from build123d import *

# Parameters (mm, degrees)
SKETCH1_W            = 98.425
SKETCH1_H            = 12.7
BOSS_EXTRUDE1_DEPTH  = 12.7
CUT_EXTRUDE1_REACH   = 54.388
SKETCH2_W            = 6.35
SKETCH2_H            = 19.05
FILLET1_R            = 3.175
FILLET2_R            = 3.175
FILLET3_R            = 3.175
FILLET4_R            = 3.175
FILLET1_OF_MIRROR1_R = 3.175
FILLET2_OF_MIRROR1_R = 3.175
FILLET3_OF_MIRROR1_R = 3.175
FILLET4_OF_MIRROR1_R = 3.175
CUT_EXTRUDE2_REACH   = 54.388
SKETCH5_W            = 55.88
SKETCH5_H            = 12.7
SKETCH6_W            = 25.4
SKETCH6_H            = 50.8
BOSS_EXTRUDE3_DEPTH  = 6.35


with BuildPart() as part:
    # Sketch1 → Boss-Extrude1 (new, symmetric)
    with BuildSketch(Plane.XY):
        Rectangle(SKETCH1_W, SKETCH1_H)
    extrude(amount=BOSS_EXTRUDE1_DEPTH, both=True)

    # Sketch2 → Cut-Extrude1 (cut, up to next)
    with BuildSketch(Plane(origin=(0, 6.35, 0), x_dir=(1, 0, 0), z_dir=(0, 1, 0)), mode=Mode.PRIVATE) as cut_extrude1_sk1:
        with Locations((-41.275, 0)):
            Rectangle(SKETCH2_W, SKETCH2_H)
    cut_extrude1_tool1 = extrude(cut_extrude1_sk1.sketch, amount=-CUT_EXTRUDE1_REACH, mode=Mode.PRIVATE) & part.part
    cut_extrude1 = cut_extrude1_tool1.solids().sort_by_distance((-41.275, 6.35, 0))[0]
    add(cut_extrude1, mode=Mode.SUBTRACT)

    # Fillet1
    fillet1_edges = [part.edges().sort_by_distance(p)[0] for p in [
        (-44.45, 0, -9.525),
    ]]
    fillet(fillet1_edges, radius=FILLET1_R)

    # Fillet2
    fillet2_edges = [part.edges().sort_by_distance(p)[0] for p in [
        (-38.1, 0, -9.525),
    ]]
    fillet(fillet2_edges, radius=FILLET2_R - 0.0001)  # a hair under: the kernel refuses the full size

    # Fillet3
    fillet3_edges = [part.edges().sort_by_distance(p)[0] for p in [
        (-44.45, 0, 9.525),
    ]]
    fillet(fillet3_edges, radius=FILLET3_R)

    # Fillet4
    fillet4_edges = [part.edges().sort_by_distance(p)[0] for p in [
        (-38.1, 0, 9.525),
    ]]
    fillet(fillet4_edges, radius=FILLET4_R - 0.0001)  # a hair under: the kernel refuses the full size

    # Mirror1: Cut-Extrude1 across plane
    add(cut_extrude1.mirror(Plane(origin=(0, 0, 0), x_dir=(0, 0, 1), z_dir=(1, 0, 0))), mode=Mode.SUBTRACT)

    # Fillet1 of Mirror1
    fillet1_of_mirror1_edges = [part.edges().sort_by_distance(p)[0] for p in [
        (44.45, 0, -9.525),
    ]]
    fillet(fillet1_of_mirror1_edges, radius=FILLET1_OF_MIRROR1_R)

    # Fillet2 of Mirror1
    fillet2_of_mirror1_edges = [part.edges().sort_by_distance(p)[0] for p in [
        (38.1, 0, -9.525),
    ]]
    fillet(fillet2_of_mirror1_edges, radius=FILLET2_OF_MIRROR1_R - 0.0001)  # a hair under: the kernel refuses the full size

    # Fillet3 of Mirror1
    fillet3_of_mirror1_edges = [part.edges().sort_by_distance(p)[0] for p in [
        (44.45, 0, 9.525),
    ]]
    fillet(fillet3_of_mirror1_edges, radius=FILLET3_OF_MIRROR1_R)

    # Fillet4 of Mirror1
    fillet4_of_mirror1_edges = [part.edges().sort_by_distance(p)[0] for p in [
        (38.1, 0, 9.525),
    ]]
    fillet(fillet4_of_mirror1_edges, radius=FILLET4_OF_MIRROR1_R - 0.0001)  # a hair under: the kernel refuses the full size

    # Sketch5 → Cut-Extrude2 (cut, up to next)
    with BuildSketch(Plane(origin=(0, 6.35, 0), x_dir=(1, 0, 0), z_dir=(0, 1, 0)), mode=Mode.PRIVATE) as cut_extrude2_sk1:
        with Locations((0, 6.35)):
            Rectangle(SKETCH5_W, SKETCH5_H)
    cut_extrude2_tool1 = extrude(cut_extrude2_sk1.sketch, amount=-CUT_EXTRUDE2_REACH, mode=Mode.PRIVATE) & part.part
    add(cut_extrude2_tool1.solids().sort_by_distance((0, 6.35, -6.35))[0], mode=Mode.SUBTRACT)

    # Sketch6 → Boss-Extrude3 (add)
    with BuildSketch(Plane(origin=(0, 0, 0), x_dir=(-1, 0, 0), z_dir=(0, 0, -1))):
        Rectangle(SKETCH6_W, SKETCH6_H)
    extrude(amount=BOSS_EXTRUDE3_DEPTH)


solid = part.part
Design review of the part built by this model. Coordinates are the model's own, in mm. A direction names the side the tool comes from. Give positions to 0.01 mm unless a question says otherwise; leave off trailing zeros. Loops run counter-clockwise (first coordinate to the right, second up) from the corner with the lowest first, then second, coordinate; pieces in that order, holes last. Notation, with made-up numbers: (76.5, 13.5) - (126.5, 13.5) arc R16 ccw to (126.5, 17.5) - close; hole circle Ø3 at (-23, 28.5). An arc over 180 degrees is marked (long way). Use CSV: the item, a comma, the result in double quotes. Start each with the question number.
1. Machinability: for faces 1 (the flat face through (0, 16, 0)), 2 (the flat face through (-44.45, 0, 0)), 3 (the flat face through (-20, 0, 0)), which of the approach directions +Z, -Z, +X, -X, +Y, -Y give a long, thin tool a straight path to every point of the face, cutting with its end or side? Answer none if there is none.
2. Draft analysis for pull direction Z (two halves, no side actions). For faces 4 (the flat face through (0, -25.4, -3)), 5 (the flat face through (-39, 0, -12.7)), 6 (the cylindrical face through (39.055, -0.089, -8.62)), 7 (the cylindrical face through (-43.545, -0.089, 8.57)), state which applies: released by +Z, released by -Z, zero draft, split by the parting line, or undercut.
3. Add section B-B (z = -1). State the section outline as (x, y) points.
4. Add section D-D (z = -7.5). State the section outline as (x, y) points, plus the area to 3 significant figures.
5. Wall thickness on L1, parallel to X at y = -4, z = 5.75; L2, parallel to Y at x = 4, z = 4; L3, parallel to X at y = -19, z = -1.5: over which ranges is each line inside the solid? List them lowest first.
6. Add section C-C (x = -6). State the section outline as (y, z) points.
7. Add section A-A (y = 2.5). Count the separate pieces of the cut face and the enclosed holes in it, plus the area to 3 significant figures.
8. Insertion check: P1, Ø5, axis at y = 9.5, z = -2, coming from the +X side; P2, Ø12.5, axis at x = 20, z = 0.5, coming from the +Y side; P3, Ø15, axis at x = 1, y = 14, coming from the +Z side; P4, Ø2, axis at y = -9, z = 7.5, coming from the +X side. Each pin has a flat end and moves straight along its axis. Give the tip position at first contact, or say it passes through.
Results found:
1,face 1,"+Z, +X, -X, +Y"
1,face 2,"+Y, -Y"
1,face 3,"-Z, +Y, -Y"
2,face 4,"zero draft"
2,face 5,"released by -Z"
2,face 6,"undercut"
2,face 7,"undercut"
3,outline,"(-49.21, -6.35) - (-44.45, -6.35) - (-44.45, 6.35) - (-49.21, 6.35) - close; (-38.1, -6.35) - (-27.94, -6.35) - (-27.94, 6.35) - (-38.1, 6.35) - close; (-12.7, -25.4) - (12.7, -25.4) - (12.7, 25.4) - (-12.7, 25.4) - close; (27.94, -6.35) - (38.1, -6.35) - (38.1, 6.35) - (27.94, 6.35) - close; (44.45, -6.35) - (49.21, -6.35) - (49.21, 6.35) - (44.45, 6.35) - close"
4,outline,"(-49.21, -6.35) - (-44.23, -6.35) - (-44.23, 6.35) - (-49.21, 6.35) - close; (-38.32, -6.35) - (-27.94, -6.35) - (-27.94, 6.35) - (-38.32, 6.35) - close; (27.94, -6.35) - (38.32, -6.35) - (38.32, 6.35) - (27.94, 6.35) - close; (44.23, -6.35) - (49.21, -6.35) - (49.21, 6.35) - (44.23, 6.35) - close"
4,area,"390 mm²"
5,L1,"x = -49.21 to -44.45, -38.1 to 38.1, 44.45 to 49.21"
5,L2,"y = -6.35 to 6.35"
5,L3,"x = -12.7 to 12.7"
6,outline,"(-25.4, -6.35) - (25.4, -6.35) - (25.4, 0) - (6.35, 0) - (6.35, 12.7) - (-6.35, 12.7) - (-6.35, 0) - (-25.4, 0) - close"
7,separate pieces,"1"
7,enclosed holes,"2"
7,area,"1,730 mm²"
8,P1,"stops at x = 12.7"
8,P2,"stops at y = 6.35"
8,P3,"stops at z = 0"
8,P4,"passes through"
